from build123d import *

# Parameters (mm, degrees)
SALIENTE_EXTRUIR1_DEPTH    = 1500
CORTAR_EXTRUIR1_DEPTH      = 10
CORTAR_EXTRUIR1_DEPTH_BACK = 40


with BuildPart() as part:
    # Croquis3 → Saliente-Extruir1 (new body)
    with BuildSketch(Plane(origin=(0, 0, 0), x_dir=(-1, 0, 0), z_dir=(0, 0, -1))):
        with BuildLine():
            Line((-4.77501925, 0), (-4.77501925, 30))
            ThreePointArc((-4.77501925, 30), (-2.653698906, 29.121320344), (-1.77501925, 27))
            Line((-1.77501925, 27), (-1.77501925, 8))
            ThreePointArc((-1.77501925, 8), (-0.310553156, 4.464466094), (3.22498075, 3))
            Line((3.22498075, 3), (22.22498075, 3))
            ThreePointArc((22.22498075, 3), (24.346301094, 2.121320344), (25.22498075, 0))
            Line((25.22498075, 0), (-4.77501925, 0))
        make_face()
    extrude(amount=-SALIENTE_EXTRUIR1_DEPTH)

    # Croquis4 → Cortar-Extruir1 (cut, two sides: drawn at the far end of the back side and taken through both)
    with BuildSketch(Plane(origin=(0, 0, 0), x_dir=(0, 0, -1), z_dir=(1, 0, 0)).offset(-CORTAR_EXTRUIR1_DEPTH_BACK)):
        Polygon((-1500, 0), (-1470, 0), (-1500, 30), align=None)
        Polygon((0, 0), (-30, 0), (0, 30), align=None)
    extrude(amount=CORTAR_EXTRUIR1_DEPTH + CORTAR_EXTRUIR1_DEPTH_BACK, mode=Mode.SUBTRACT)


solid = part.part
Verification items for the finished model (mm, model axes). Give positions to 0.01 mm unless a question says otherwise; leave off trailing zeros. Loops run counter-clockwise (first coordinate to the right, second up) from the corner with the lowest first, then second, coordinate; pieces in that order, holes last.
1. Cross-section at B-B on y = 15. Record the cut outline in (x, z).
Derived:
outline: (1.78, 15) - (4.78, 15) - (4.78, 1485) - (1.78, 1485) - close
2. Material ranges on probe 1 along Y at (x, z) = (-9, 344); probe 2 along X at (y, z) = (12, 119); probe 3 along X at (y, z) = (7.5, 801), recorded low to high.
Derived:
probe 1: y = 0 to 3
probe 2: x = 1.78 to 4.78
probe 3: x = 1.75 to 4.78
3. Cross-section at C-C on x = -15. Record the cut outline in (y, z), and give its area (3 significant figures).
Derived:
outline: (0, 30) - (3, 27) - (3, 1473) - (0, 1470) - close
area: 4,330 mm2
4. Cross-section at A-A on z = 121. Record the cut outline in (x, y), and give its area (3 significant figures).
Derived:
outline: (-25.22, 0) - (4.78, 0) - (4.78, 30) arc R3 ccw to (1.78, 27) - (1.78, 8) arc R5 cw to (-3.22, 3) - (-22.22, 3) arc R3 ccw to start
area: 173 mm2
5. Go/stop test with flat-tipped pins: P1, Ø5, axis at x = -6, z = 347.5, coming from the +Y side; P2, Ø12, axis at x = -7.5, z = 1137, coming from the +Y side; P3, Ø15, axis at y = 21, z = 741.5, coming from the -X side (3 decimals); P4, Ø12, axis at x = 1.5, y = 25.5, coming from the +Z side. Record where each tip stops, or that it passes through.
Derived:
P1: stops at y = 3
P2: stops at y = 3.31
P3: stops at x = 1.775
P4: stops at z = 1500
